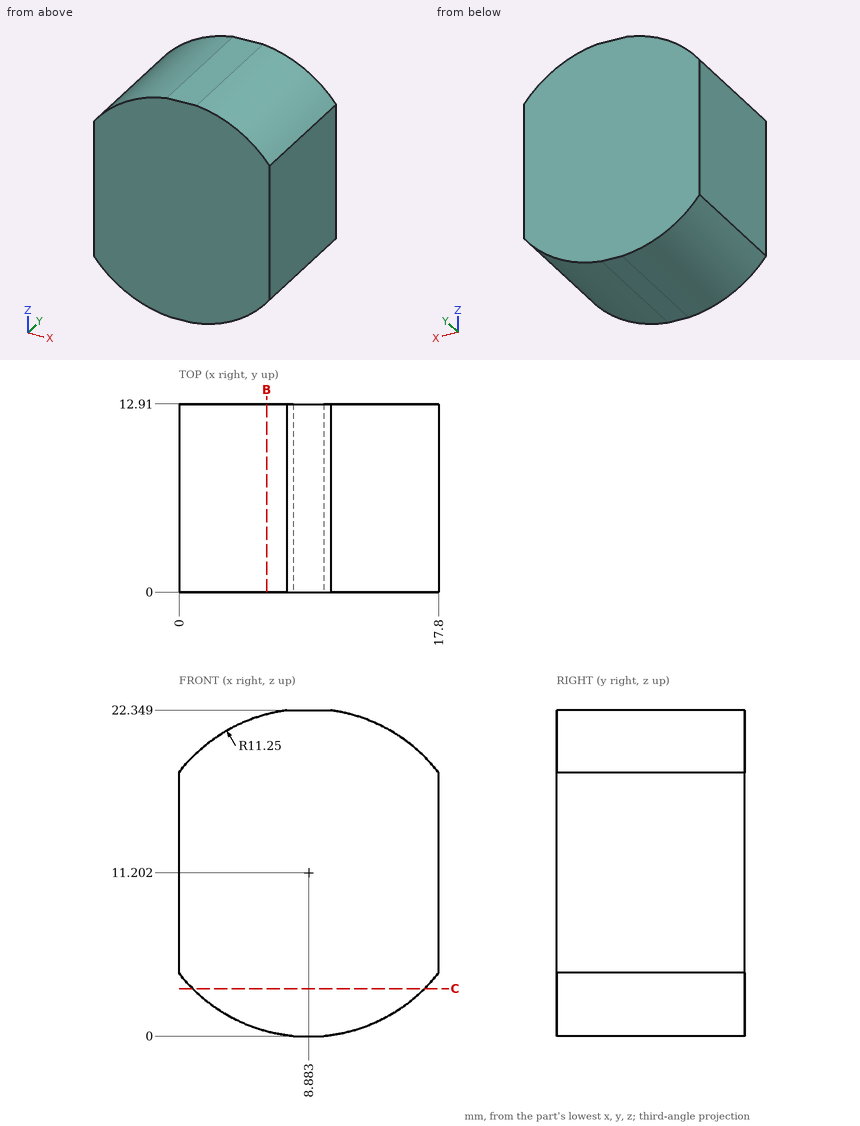
Study the drawing (mm; zero at the part's minimum x, y, z) and answer. Round coordinates to 2 decimals unless told otherwise and drop trailing zeros. Order: outer loops, then holes, each group sorted by start corner. A loop starts at its lowest first (then second) coordinate and runs counter-clockwise, first axis right, second up. Notation, with made-up numbers: (15, 69.5) -> (50, 69.5) arc R9 cw to (50, 78.5) -> close; hole circle Ø9 at (-20.5, -24). An arc over 180 degrees is marked (long way). Write each question's results on one line, items separated by ' | '. Start each with the question number.
Q1. Find section B-B (x = 6). Determine the outline of the cut face in (y, z), then the cut area to 3 significant figures.
Q2. Find section C-C (z = 3.25). Determine the outline of the cut face in (x, y) (3 decimals).
Q3. Straight lines are drawn through the part: probe 1 along X at (y, z) = (1, 20.75) (1 decimal); probe 2 along Z at (x, y) = (12.5, 4.75) (1 decimal); probe 3 along Z at (x, y) = (12, 1.75). For each, find the intervals that lie inside material, in ascending order. Write a range as from..to.
Worked answers:
1) outline: (0, 0.33) -> (12.91, 0.33) -> (12.91, 22.08) -> (0, 22.08) -> close | area: 281 mm2
2) outline: (0.925, 0) -> (16.841, 0) -> (16.841, 12.91) -> (0.925, 12.91) -> close
3) probe 1: x = 2.9..14.8 | probe 2: z = 0.5..21.9 | probe 3: z = 0.39..22.01
